from build123d import *
from build123d import SkipClean  # not in build123d's __all__

# Parameters (mm, degrees)
F0_R     = 5
F1_DEPTH = 8
F3_DEPTH = 20
F4_DEPTH = 20.001
F5_DEPTH = 4


with BuildPart() as f1:
    # F0 (on Top) → F1 (new body)
    with BuildSketch(Plane.XY):
        with BuildLine():
            Line((-19, -10), (19, -10))
            ThreePointArc((19, -10), (29, 0), (19, 10))
            Line((19, 10), (-19, 10))
            ThreePointArc((-19, 10), (-29, 0), (-19, -10))
        make_face()
        with Locations((-19, 0)):
            Circle(F0_R, mode=Mode.SUBTRACT)
        with Locations((19, 0)):
            Circle(F0_R, mode=Mode.SUBTRACT)
    extrude(amount=F1_DEPTH)

    # F2 (on face) → F3 (join, through all)
    with BuildSketch(Plane.XZ.offset(10)):
        with BuildLine():
            Line((-10, 11), (-10, 8))
            Line((-10, 8), (-6.3245553203, 8))
            ThreePointArc((-6.3245553203, 8), (-1.5375488216, 17.8290514437), (7, 11))
            ThreePointArc((7, 11), (6.8290514437, 9.4624511784), (6.3245553203, 8))
            Line((6.3245553203, 8), (10, 8))
            Line((10, 8), (10, 11))
            ThreePointArc((10, 11), (0, 21), (-10, 11))
        make_face()
        with BuildLine():
            Line((-4, 8), (-6.3245553203, 8))
            ThreePointArc((-6.3245553203, 8), (0, 4), (6.3245553203, 8))
            Line((6.3245553203, 8), (4, 8))
            ThreePointArc((4, 8), (0, 6), (-4, 8))
        make_face()
        with BuildLine():
            ThreePointArc((7, 11), (-1.5375488216, 17.8290514437), (-6.3245553203, 8))
            Line((-6.3245553203, 8), (-4, 8))
            ThreePointArc((-4, 8), (-1.5811388301, 15.7434164903), (5, 11))
            ThreePointArc((5, 11), (4.7434164903, 9.4188611699), (4, 8))
            Line((4, 8), (6.3245553203, 8))
            ThreePointArc((6.3245553203, 8), (6.8290514437, 9.4624511784), (7, 11))
        make_face()
    extrude(amount=-F3_DEPTH)

    # F2 (on face) → F4 (cut, through all)
    with BuildSketch(Plane.XZ.offset(10)):
        with BuildLine():
            Line((4, 8), (-4, 8))
            ThreePointArc((-4, 8), (0, 6), (4, 8))
        make_face()
    with SkipClean():  # cleaning this boolean's faces spoils the solid; the shape is the same uncleaned
        extrude(amount=-F4_DEPTH, mode=Mode.SUBTRACT)

    # F2 (on face) → F5 (join)
    with BuildSketch(Plane.XZ.offset(10)):
        with BuildLine():
            Line((-4, 8), (-6.3245553203, 8))
            ThreePointArc((-6.3245553203, 8), (0, 4), (6.3245553203, 8))
            Line((6.3245553203, 8), (4, 8))
            ThreePointArc((4, 8), (0, 6), (-4, 8))
        make_face()
        with BuildLine():
            ThreePointArc((7, 11), (-1.5375488216, 17.8290514437), (-6.3245553203, 8))
            Line((-6.3245553203, 8), (-4, 8))
            ThreePointArc((-4, 8), (-1.5811388301, 15.7434164903), (5, 11))
            ThreePointArc((5, 11), (4.7434164903, 9.4188611699), (4, 8))
            Line((4, 8), (6.3245553203, 8))
            ThreePointArc((6.3245553203, 8), (6.8290514437, 9.4624511784), (7, 11))
        make_face()
    extrude(amount=F5_DEPTH)


solid = f1.part
Can you work these out from the model? Positions are in its coordinate system, mm. A direction names the side the tool comes from. Coordinates: 2 decimals unless noted, no trailing zeros. Loops run counter-clockwise (first coordinate to the right, second up) from the corner with the lowest first, then second, coordinate; pieces in that order, holes last. Notation, with made-up numbers: (45.5, 55.25) - (75.5, 55.25) arc R23 ccw to (75.5, 65.25) - close; hole circle Ø1 at (20, -36). An arc over 180 degrees is marked (long way). Answer as a JSON object with one key per item and string values. Group by question number.
Item 1: If we section it at B-B (x = -1): List the corners of the cut face in (y, z) for me, plus the area to 3 significant figures.
Item 2: If we section it at C-C (y = -11.5): List the corners of the cut face in (x, z) for me, plus the area to 3 significant figures.
Item 3: If we mould it in two halves opening along Y, with no side actions, what happens to faces 4 (the face through (-0.3, -10, 3.6)), 5 (the face through (29, 0, 4)), 6 (the face through (21, 5, 8)), 7 (the face through (14, 0, 4))? For each: released by +Y, released by -Y, zero draft, split by the parting line, or undercut.
Item 4: If I drill on L1, parallel to X at y = -10.85, z = 11; L2, parallel to X at y = -2.25, z = 4.5; L3, parallel to Y at x = 19, z = 5.75, over which ranges is the centre line in solid material (lowest first)? Write a range as from..to.
Item 5: If we section it at D-D (z = 11.75): List the corners of the cut face in (x, y) for me, plus the area to 3 significant figures.
Item 6: If we section it at A-A (y = 0): List the corners of the cut face in (x, z) for me, plus the area to 3 significant figures.
Item 7: For pin 1 (6 mm diameter, centred on y = 5.5, z = 12, fed in from +X); pin 2 (4 mm diameter, centred on y = 1.5, z = 17.5, fed in from +X); pin 3 (5 mm diameter, centred on x = -4, y = -8.5, fed in from +Z), each with a flat end and sliding along its axis, tell me the tip position at first contact or that it passes through.
Item 8: On a 3-axis mill with a long thin cutter (end or side, diameter ignored), from which of +Z, -Z, +X, -X, +Y, -Y can I reach the whole of each face in a straight line? I mean faces 1 (the face through (10, 0, 9)), 2 (the face through (0, 0, 21)), 3 (the face through (-10, 0, 10)). Say none if no direction works.
Returned:
{
 "1": {"outline": "(-14, 4.07) - (-10, 4.07) - (-10, 0) - (10, 0) - (10, 6.1) - (-14, 6.1) - close; (-14, 15.9) - (10, 15.9) - (10, 20.95) - (-10, 20.95) - (-10, 17.93) - (-14, 17.93) - close", "area": "239 mm²"},
 "2": {"outline": "circle Ø14 at (0, 11); hole circle Ø10 at (0, 11)", "area": "75.4 mm²"},
 "3": {"face 4": "released by -Y", "face 5": "split by the parting line", "face 6": "zero draft", "face 7": "undercut"},
 "4": {"L1": "x = -7..-5, 5..7", "L2": "x = -28.74..-23.47, -14.53..14.53, 23.47..28.74", "L3": "y = -10..-5, 5..10"},
 "5": {"outline": "(-9.97, -10) - (-6.96, -10) - (-6.96, -14) - (-4.94, -14) - (-4.94, 10) - (-9.97, 10) - close; (4.94, -14) - (6.96, -14) - (6.96, -10) - (9.97, -10) - (9.97, 10) - (4.94, 10) - close", "area": "217 mm²"},
 "6": {"outline": "(-29, 0) - (-24, 0) - (-24, 8) - (-29, 8) - close; (-14, 0) - (14, 0) - (14, 8) - (10, 8) - (10, 11) arc R10 ccw to (-10, 11) - (-10, 8) - (-14, 8) - close; (24, 0) - (29, 0) - (29, 8) - (24, 8) - close; hole circle Ø10 at (0, 11)", "area": "443 mm²"},
 "7": {"pin 1": "stops at x = 10", "pin 2": "stops at x = 8.93", "pin 3": "stops at z = 20.89"},
 "8": {"face 1": "+Z, +X, +Y, -Y", "face 2": "+Z, +Y, -Y", "face 3": "+Z, -X, +Y, -Y"}
}
